Design review of the part built by this model. Coordinates are the model's own, in mm. Give positions to 0.01 mm unless a question says otherwise; leave off trailing zeros. Order: outer loops, then holes, each group sorted by start corner. A loop starts at its lowest first (then second) coordinate and runs counter-clockwise, first axis right, second up. Notation, with made-up numbers: (51, -12) -> (87, -12) arc R30 cw to (87, 10) -> close; hole circle Ø2 at (20, 2). An arc over 180 degrees is marked (long way). Answer in a Markdown table with one row per item. Add a question column.
```python
from build123d import *

# Parameters (mm, degrees)
F0_R     = 155.575
F0_R_2   = 12.7
F1_DEPTH = 3.175


with BuildPart() as f1:
    # F0 (on Top) → F1 (new body)
    with BuildSketch(Plane.XY):
        Circle(F0_R)
        with BuildLine():
            Line((-1.5875, -15.795426), (-1.5875, -152.391732))
            ThreePointArc((-1.5875, -152.391732), (-107.763073, -107.763073), (-152.391732, -1.5875))
            Line((-152.391732, -1.5875), (-15.795426, -1.5875))
            ThreePointArc((-15.795426, -1.5875), (-11.22532, -11.22532), (-1.5875, -15.795426))
        make_face(mode=Mode.SUBTRACT)
        with BuildLine():
            ThreePointArc((152.391732, -1.5875), (107.763073, -107.763073), (1.5875, -152.391732))
            Line((1.5875, -152.391732), (1.5875, -15.795426))
            ThreePointArc((1.5875, -15.795426), (11.22532, -11.22532), (15.795426, -1.5875))
            Line((15.795426, -1.5875), (152.391732, -1.5875))
        make_face(mode=Mode.SUBTRACT)
        with BuildLine():
            ThreePointArc((-152.391732, 1.5875), (-107.763073, 107.763073), (-1.5875, 152.391732))
            Line((-1.5875, 152.391732), (-1.5875, 15.795426))
            ThreePointArc((-1.5875, 15.795426), (-11.22532, 11.22532), (-15.795426, 1.5875))
            Line((-15.795426, 1.5875), (-152.391732, 1.5875))
        make_face(mode=Mode.SUBTRACT)
        Circle(F0_R_2, mode=Mode.SUBTRACT)
        with BuildLine():
            Line((1.5875, 15.795426), (1.5875, 152.391732))
            ThreePointArc((1.5875, 152.391732), (107.763073, 107.763073), (152.391732, 1.5875))
            Line((152.391732, 1.5875), (15.795426, 1.5875))
            ThreePointArc((15.795426, 1.5875), (11.22532, 11.22532), (1.5875, 15.795426))
        make_face(mode=Mode.SUBTRACT)
    extrude(amount=F1_DEPTH)


solid = f1.part
```
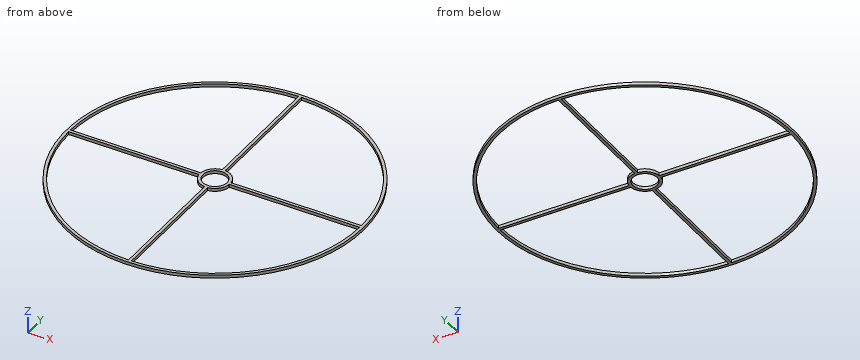
1) Add section B-B, the plane z = 1.6. Give the number of separate pieces and of enclosed holes in the cut face, and give its area (3 significant figures).
2) Clearance check with flat-ended pins moving along their axes: P1, Ø1, axis at y = -81, z = 1.5, coming from the +X side; P2, Ø1, axis at y = -63.5, z = 2, coming from the -X side; P3, Ø1, axis at x = 84, z = 1.5, coming from the -Y side. State where each tip first meets the part, or that it passes through.
3) Add section A-A, the plane x = 20. Write out the cut boundary in (y, z) (1 decimal), and give its area (3 significant figures).
4) For L1, parallel to X at y = -74, z = 0.65; L2, parallel to Y at x = 0, z = 2.35 (3 decimals); L3, parallel to X at y = 71.5, z = 0.55, list the stretches that pass through material, from the lowest coordinate up.
5) Add section C-C, the plane y = -134. Write out the cut boundary in (x, z) (1 decimal).
Verdict:
| question | item | result |
|---|---|---|
| 1 | separate pieces | 1 |
| 1 | enclosed holes | 5 |
| 1 | area | 5,090 mm2 |
| 2 | P1 | stops at x = 133.13 |
| 2 | P2 | stops at x = -142.25 |
| 2 | P3 | stops at y = -131.27 |
| 3 | outline | (-154.3, 0) -> (-151.1, 0) -> (-151.1, 3.2) -> (-154.3, 3.2) -> close; (-1.6, 0) -> (1.6, 0) -> (1.6, 3.2) -> (-1.6, 3.2) -> close; (151.1, 0) -> (154.3, 0) -> (154.3, 3.2) -> (151.1, 3.2) -> close |
| 3 | area | 30.4 mm2 |
| 4 | L1 | x = -136.85 to -133.23, -1.59 to 1.59, 133.23 to 136.85 |
| 4 | L2 | y = -155.575 to -12.7, 12.7 to 155.575 |
| 4 | L3 | x = -138.17 to -134.59, -1.59 to 1.59, 134.59 to 138.17 |
| 5 | outline | (-79, 0) -> (-72.6, 0) -> (-72.6, 3.2) -> (-79, 3.2) -> close; (-1.6, 0) -> (1.6, 0) -> (1.6, 3.2) -> (-1.6, 3.2) -> close; (72.6, 0) -> (79, 0) -> (79, 3.2) -> (72.6, 3.2) -> close |
